```python
from build123d import *

# Parameters (mm, degrees)
SKETCH_1_W           = 80
SKETCH_1_H           = 97
EXTRUDE_1_DEPTH      = 22
EXTRUDE_1_DEPTH_BACK = 22
SKETCH_2_R           = 3
EXTRUDE_2_DEPTH      = 6
CUT_EXTRUDE_1_DEPTH  = 116
SKETCH_4_R           = 19
SKETCH_4_R_2         = 4
EXTRUDE_3_DEPTH      = 5
SKETCH_5_R           = 2.6
SKETCH_5_R_2         = 4
EXTRUDE_4_DEPTH      = 10
SKETCH_6_R           = 4
CUT_EXTRUDE_2_DEPTH  = 28


with BuildPart() as part:
    # Sketch 1 → Extrude 1 (new body, two sides)
    with BuildSketch(Plane.XY) as extrude_1_sk:
        with Locations((10.184545044, -4.84675016)):
            Rectangle(SKETCH_1_W, SKETCH_1_H)
    extrude(amount=EXTRUDE_1_DEPTH)
    extrude(extrude_1_sk.sketch, amount=-EXTRUDE_1_DEPTH_BACK)

    # Sketch 2 → Extrude 2 (add)
    with BuildSketch(Plane.XY.offset(22)):
        with BuildLine():
            Line((5.696739445, -50.577243051), (3.963993083, -40.133962282))
            ThreePointArc((3.963993083, -40.133962282), (-9.260891439, -32.792186642), (-16.602667079, -19.56730212))
            Line((-16.602667079, -19.56730212), (-27.045947847, -17.834555759))
            ThreePointArc((-27.045947847, -17.834555759), (-27.315454956, -13.34675016), (-27.045947847, -8.858944561))
            Line((-27.045947847, -8.858944561), (-16.602667079, -7.126198199))
            ThreePointArc((-16.602667079, -7.126198199), (-9.260891439, 6.098686323), (3.963993083, 13.440461963))
            Line((3.963993083, 13.440461963), (5.696739445, 23.883742731))
            ThreePointArc((5.696739445, 23.883742731), (10.184545044, 24.15324984), (14.672350643, 23.883742731))
            Line((14.672350643, 23.883742731), (16.405097004, 13.440461963))
            ThreePointArc((16.405097004, 13.440461963), (29.629981526, 6.098686323), (36.971757166, -7.126198199))
            Line((36.971757166, -7.126198199), (47.415037935, -8.858944561))
            ThreePointArc((47.415037935, -8.858944561), (47.684545044, -13.34675016), (47.415037935, -17.834555759))
            Line((47.415037935, -17.834555759), (36.971757166, -19.56730212))
            ThreePointArc((36.971757166, -19.56730212), (29.629981526, -32.792186642), (16.405097004, -40.133962282))
            Line((16.405097004, -40.133962282), (14.672350643, -50.577243051))
            ThreePointArc((14.672350643, -50.577243051), (10.184545044, -50.84675016), (5.696739445, -50.577243051))
        make_face()
        with Locations((10.184545044, -45.84675016)):
            Circle(SKETCH_2_R, mode=Mode.SUBTRACT)
        with Locations((-22.315454956, -13.34675016)):
            Circle(SKETCH_2_R, mode=Mode.SUBTRACT)
        with Locations((10.184545044, 19.15324984)):
            Circle(SKETCH_2_R, mode=Mode.SUBTRACT)
        with Locations((42.684545044, -13.34675016)):
            Circle(SKETCH_2_R, mode=Mode.SUBTRACT)
    extrude_2 = extrude(amount=EXTRUDE_2_DEPTH)

    # Mirror 1: Extrude 2 across plane
    add(extrude_2.mirror(Plane.XY))

    # Sketch 3 → Cut-Extrude 1 (cut)
    with BuildSketch(Plane.XY.offset(28)):
        with BuildLine():
            Line((7.568069443, -6.854134706), (7.568069443, -3.854134706))
            Line((7.568069443, -3.854134706), (12.801020645, -3.854134706))
            Line((12.801020645, -3.854134706), (12.801020645, -6.854134706))
            ThreePointArc((12.801020645, -6.854134706), (10.184545044, -20.34675016), (7.568069443, -6.854134706))
        make_face()
    extrude(amount=-CUT_EXTRUDE_1_DEPTH, mode=Mode.SUBTRACT)

    # Sketch 4 → Extrude 3 (add)
    with BuildSketch(Plane.ZY.offset(29.815454956)):
        with Locations((0, 16.65324984)):
            Circle(SKETCH_4_R)
        with Locations((0, 16.65324984)):
            Circle(SKETCH_4_R_2, mode=Mode.SUBTRACT)
    extrude(amount=EXTRUDE_3_DEPTH)

    # Sketch 5 → Extrude 4 (add)
    with BuildSketch(Plane.ZY.offset(34.815454956)):
        with BuildLine():
            Line((-26, 46.65324984), (26, 46.65324984))
            ThreePointArc((26, 46.65324984), (27.414213562, 46.067463403), (28, 44.65324984))
            Line((28, 44.65324984), (28, -11.34675016))
            ThreePointArc((28, -11.34675016), (27.414213562, -12.760963722), (26, -13.34675016))
            Line((26, -13.34675016), (-26, -13.34675016))
            ThreePointArc((-26, -13.34675016), (-27.414213562, -12.760963722), (-28, -11.34675016))
            Line((-28, -11.34675016), (-28, 44.65324984))
            ThreePointArc((-28, 44.65324984), (-27.414213562, 46.067463403), (-26, 46.65324984))
        make_face()
        with Locations((23.5, 40.15324984)):
            Circle(SKETCH_5_R, mode=Mode.SUBTRACT)
        with Locations((-23.5, 40.15324984)):
            Circle(SKETCH_5_R, mode=Mode.SUBTRACT)
        with Locations((23.5, -6.84675016)):
            Circle(SKETCH_5_R, mode=Mode.SUBTRACT)
        with Locations((-23.5, -6.84675016)):
            Circle(SKETCH_5_R, mode=Mode.SUBTRACT)
        with Locations((0, 16.65324984)):
            Circle(SKETCH_5_R_2, mode=Mode.SUBTRACT)
    extrude(amount=EXTRUDE_4_DEPTH)

    # Sketch 6 → Cut-Extrude 2 (cut)
    with BuildSketch(Plane.ZY.offset(29.815454956)):
        with Locations((0, 16.65324984)):
            Circle(SKETCH_6_R)
    extrude(amount=-CUT_EXTRUDE_2_DEPTH, mode=Mode.SUBTRACT)


solid = part.part
```
Verification items for the finished model (mm, model axes). A direction names the side the tool comes from. Coordinates: 2 decimals unless noted, no trailing zeros. Loops run counter-clockwise (first coordinate to the right, second up) from the corner with the lowest first, then second, coordinate; pieces in that order, holes last. Notation, with made-up numbers: (62.25, -36.75) -> (77.25, -36.75) arc R8 cw to (77.25, -32.75) -> close; hole circle Ø10 at (49.25, 10). An arc over 180 degrees is marked (long way). Answer in a Markdown table with one row per item.
1) Draft check along X on faces 4 (the face through (11, -21, 28)), 5 (the face through (10, -46, -22)), 6 (the face through (15.527, 18.735, 24.958)). Enter one of: released by +X, released by -X, zero draft, split by the parting line, or undercut.
The answers:
| item | result |
|---|---|
| face 4 | zero draft |
| face 5 | undercut |
| face 6 | released by +X |
2) Section check D-D (z = 23.5). Give the number of separate pieces and of enclosed holes in the cut face, and give its area (3 significant figures).
The answers:
| item | result |
|---|---|
| separate pieces | 4 |
| enclosed holes | 5 |
| area | 3,020 mm2 |
3) Section check A-A (z = 0). Record the cut outline in (x, y), and give its area (3 significant figures).
The answers:
| item | result |
|---|---|
| outline | (-44.82, -13.35) -> (-34.82, -13.35) -> (-34.82, -2.35) -> (-29.82, -2.35) -> (-29.82, -53.35) -> (50.18, -53.35) -> (50.18, 43.65) -> (-29.82, 43.65) -> (-29.82, 35.65) -> (-34.82, 35.65) -> (-34.82, 46.65) -> (-44.82, 46.65) -> (-44.82, 20.65) -> (-1.82, 20.65) -> (-1.82, 12.65) -> (-44.82, 12.65) -> close; hole (7.57, -6.85) arc R7 ccw (long way) to (12.8, -6.85) -> (12.8, -3.85) -> (7.57, -3.85) -> close |
| area | 8,040 mm2 |
4) Scan lines: line 1 along Y through (x, z) = (-38, 23.5); line 2 along Y through (x, z) = (-39, 23); line 3 along X through (y, z) = (-7, -7). Record each from-to range of solid material in increasing order. Write a range as from..to.
The answers:
| item | result |
|---|---|
| line 1 | y = -13.35..-9.45, -4.25..37.55, 42.75..46.65 |
| line 2 | y = -13.35..-9.4, -4.3..37.6, 42.7..46.65 |
| line 3 | x = -44.82..-34.82, -29.82..7.23, 13.14..50.18 |
5) Depth check by flat-ended pin: P1, Ø4, axis at y = 16, z = -0.5, coming from the -X side; P2, Ø22, axis at x = 12, z = -8.5, coming from the +Y side; P3, Ø4, axis at y = -6.85, z = 23.5, coming from the -X side. Enter the tip coordinate at first touch or a pass-through.
The answers:
| item | result |
|---|---|
| P1 | stops at x = -1.82 |
| P2 | stops at y = 43.65 |
| P3 | stops at x = -29.82 |
6) Section check B-B (x = -5). Record the cut outline in (y, z).
The answers:
| item | result |
|---|---|
| outline | (-53.35, -22) -> (-36.27, -22) -> (-36.27, -28) -> (9.58, -28) -> (9.58, -22) -> (43.65, -22) -> (43.65, 22) -> (9.58, 22) -> (9.58, 28) -> (-36.27, 28) -> (-36.27, 22) -> (-53.35, 22) -> close; hole circle Ø8 at (16.65, 0) |
7) Section check C-C (y = 3). Record the cut outline in (x, z).
The answers:
| item | result |
|---|---|
| outline | (-44.82, -28) -> (-34.82, -28) -> (-34.82, -13.21) -> (-29.82, -13.21) -> (-29.82, -22) -> (-11.93, -22) -> (-11.93, -28) -> (32.3, -28) -> (32.3, -22) -> (50.18, -22) -> (50.18, 22) -> (32.3, 22) -> (32.3, 28) -> (-11.93, 28) -> (-11.93, 22) -> (-29.82, 22) -> (-29.82, 13.21) -> (-34.82, 13.21) -> (-34.82, 28) -> (-44.82, 28) -> close |
8) Access from +Z, -Z, +X, -X, +Y, -Y to the whole of each face (thin tool, end or side, straight path). Record for faces 1 (the face through (10.248, -50.847, 24.958)), 2 (the face through (-39.75, 40.93, 25.98)), 3 (the face through (-32.28, 22.36, 18.123)).
The answers:
| item | result |
|---|---|
| face 1 | +Z, -Y |
| face 2 | -X |
| face 3 | none |
